Input: part model. Units: mm. Frame: model coordinates. Coordinates: 2 decimals unless noted, no trailing zeros. Order: outer loops, then holes, each group sorted by start corner. A loop starts at its lowest first (then second) coordinate and runs counter-clockwise, first axis right, second up. Notation, with made-up numbers: M 30.25,25 L 68.25,25 A14 ccw 68.25,39 Z; hole C 27.5,64 d8. An arc over 180 degrees is marked long. Answer in a Markdown table with one row per item.
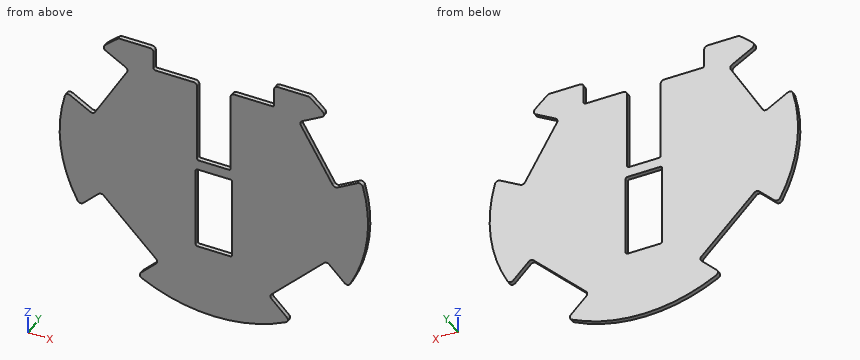
from build123d import *

# Parameters (mm, degrees)
RESSALTO_EXTRUS_O1_DEPTH = 2.5
ESBO_O13_W               = 20.5
ESBO_O13_H               = 48
CORTE_EXTRUS_O8_DEPTH    = 124.061976256
FILETE1_R                = 2
FILETE2_R                = 1


# Read off the part's stored shape, not the designer's step: Ressalto-extrusão1
with BuildPart() as part:
    # Ressalto-extrusão1 outline → Ressalto-extrusão1 (new body)
    with BuildSketch(Plane(origin=(0, 0, 0), x_dir=(1, 0, 0), z_dir=(0, 1, 0))):
        with BuildLine():
            ThreePointArc((41.182170498, 73.709082433), (41.745717904, 75.420720863), (40.703673569, 76.89090296))
            ThreePointArc((40.703673569, 76.89090296), (0, 87), (-40.703673569, 76.89090296))
            ThreePointArc((-40.703673569, 76.89090296), (-41.745717904, 75.420720863), (-41.182170498, 73.709082433))
            Line((-41.182170498, 73.709082433), (-32.526911935, 65.053823869))
            ThreePointArc((-32.526911935, 65.053823869), (-31.941125497, 63.639610306), (-32.526911935, 62.225396744))
            Line((-32.526911935, 62.225396744), (-62.225396744, 32.526911935))
            ThreePointArc((-62.225396744, 32.526911935), (-63.639610306, 31.941125497), (-65.053823869, 32.526911935))
            Line((-65.053823869, 32.526911935), (-73.709082433, 41.182170498))
            ThreePointArc((-73.709082433, 41.182170498), (-75.420720863, 41.745717904), (-76.89090296, 40.703673569))
            ThreePointArc((-76.89090296, 40.703673569), (-86.449685697, 9.769945899), (-84.035651423, -22.516866789))
            ThreePointArc((-84.035651423, -22.516866789), (-82.869168521, -23.846994955), (-81.103797367, -23.731288475))
            Line((-81.103797367, -23.731288475), (-69.755752861, -17.179491924))
            ThreePointArc((-69.755752861, -17.179491924), (-68.238114771, -16.979691079), (-67.023702054, -17.911542732))
            Line((-67.023702054, -17.911542732), (-49.023702054, -49.088457268))
            ThreePointArc((-49.023702054, -49.088457268), (-48.823901209, -50.606095358), (-49.755752861, -51.820508076))
            Line((-49.755752861, -51.820508076), (-61.103797367, -58.372304626))
            ThreePointArc((-61.103797367, -58.372304626), (-62.086687696, -59.843307652), (-61.518004364, -61.518575561))
            ThreePointArc((-61.518004364, -61.518575561), (-57.944854795, -64.895252544), (-54.186675605, -68.064705882))
            ThreePointArc((-54.186675605, -68.064705882), (-53.600773132, -68.388042871), (-52.941004902, -68.5))
            Line((-52.941004902, -68.5), (52.941004902, -68.5))
            ThreePointArc((52.941004902, -68.5), (53.600773132, -68.388042871), (54.186675605, -68.064705882))
            ThreePointArc((54.186675605, -68.064705882), (57.944854795, -64.895252544), (61.518004364, -61.518575561))
            ThreePointArc((61.518004364, -61.518575561), (62.086687696, -59.843307652), (61.103797367, -58.372304626))
            Line((61.103797367, -58.372304626), (49.755752861, -51.820508076))
            ThreePointArc((49.755752861, -51.820508076), (48.823901209, -50.606095358), (49.023702054, -49.088457268))
            Line((49.023702054, -49.088457268), (67.023702054, -17.911542732))
            ThreePointArc((67.023702054, -17.911542732), (68.238114771, -16.979691079), (69.755752861, -17.179491924))
            Line((69.755752861, -17.179491924), (81.103797367, -23.731288475))
            ThreePointArc((81.103797367, -23.731288475), (82.869168521, -23.846994955), (84.035651423, -22.516866789))
            ThreePointArc((84.035651423, -22.516866789), (86.449685697, 9.769945899), (76.89090296, 40.703673569))
            ThreePointArc((76.89090296, 40.703673569), (75.420720863, 41.745717904), (73.709082433, 41.182170498))
            Line((73.709082433, 41.182170498), (65.053823869, 32.526911935))
            ThreePointArc((65.053823869, 32.526911935), (63.639610306, 31.941125497), (62.225396744, 32.526911935))
            Line((62.225396744, 32.526911935), (32.526911935, 62.225396744))
            ThreePointArc((32.526911935, 62.225396744), (31.941125497, 63.639610306), (32.526911935, 65.053823869))
            Line((32.526911935, 65.053823869), (41.182170498, 73.709082433))
        make_face()
    extrude(amount=RESSALTO_EXTRUS_O1_DEPTH)

    # Esboço13 → Corte-extrusão8 (cut, through all)
    with BuildSketch(Plane.XZ):
        with BuildLine():
            ThreePointArc((-9.5, 67.5), (-9.207106781, 68.207106781), (-8.5, 68.5))
            Line((-8.5, 68.5), (-34, 68.5))
            Line((-34, 68.5), (-34, 55.5))
            Line((-34, 55.5), (-9.5, 55.5))
            Line((-9.5, 55.5), (-9.5, 67.5))
        make_face()
        with BuildLine():
            Line((34, 68.5), (8.5, 68.5))
            ThreePointArc((8.5, 68.5), (9.207106781, 68.207106781), (9.5, 67.5))
            Line((9.5, 67.5), (9.5, 55.5))
            Line((9.5, 55.5), (34, 55.5))
            Line((34, 55.5), (34, 68.5))
        make_face()
        with BuildLine():
            Line((8.5, 68.5), (-8.5, 68.5))
            ThreePointArc((-8.5, 68.5), (-9.207106781, 68.207106781), (-9.5, 67.5))
            Line((-9.5, 67.5), (-9.5, 55.5))
            Line((-9.5, 55.5), (9.5, 55.5))
            Line((9.5, 55.5), (9.5, 67.5))
            ThreePointArc((9.5, 67.5), (9.207106781, 68.207106781), (8.5, 68.5))
        make_face()
        with BuildLine():
            Line((9.5, 55.5), (-9.5, 55.5))
            Line((-9.5, 55.5), (-9.5, 8.5))
            ThreePointArc((-9.5, 8.5), (-9.207106781, 7.792893219), (-8.5, 7.5))
            Line((-8.5, 7.5), (8.5, 7.5))
            ThreePointArc((8.5, 7.5), (9.207106781, 7.792893219), (9.5, 8.5))
            Line((9.5, 8.5), (9.5, 55.5))
        make_face()
        with Locations((0, -22.35)):
            Rectangle(ESBO_O13_W, ESBO_O13_H)
    extrude(amount=-CORTE_EXTRUS_O8_DEPTH, mode=Mode.SUBTRACT)

    # Filete1
    filete1_edges = [part.edges().sort_by_distance(p)[0] for p in [
        (-9.5, 1.25, 55.5),
        (-34, 1.25, 68.5),
        (34, 1.25, 68.5),
        (9.5, 1.25, 55.5),
    ]]
    fillet(filete1_edges, radius=FILETE1_R)

    # Filete2
    filete2_edges = [part.edges().sort_by_distance(p)[0] for p in [
        (-34, 1.25, 55.5),
        (34, 1.25, 55.5),
        (-10.25, 1.25, 1.65),
        (10.25, 1.25, 1.65),
        (10.25, 1.25, -46.35),
        (-10.25, 1.25, -46.35),
    ]]
    fillet(filete2_edges, radius=FILETE2_R)


solid = part.part
1) Cut plane D-D, the plane x = 26.5. Output: boundary loops of the cut face in (y, z).
Resolved:
| item | result |
|---|---|
| outline | M 0,-82.87 L 2.5,-82.87 L 2.5,55.5 L 0,55.5 Z |
2) Cut plane B-B, the plane z = -20.5. Output: boundary loops of the cut face in (x, y).
Resolved:
| item | result |
|---|---|
| outline | M -84.55,0 L -10.25,0 L -10.25,2.5 L -84.55,2.5 Z; M 10.25,0 L 84.55,0 L 84.55,2.5 L 10.25,2.5 Z |
3) Contact query for flat-ended pins moving along their axis: pin 1 (10 mm diameter, centred on x = 32.5, z = -58, fed in from -Y); pin 2 (1.5 mm diameter, centred on x = 2, y = 1, fed in from +Z); pin 3 (1.2 mm diameter, centred on y = 1.5, z = 23.5, fed in from +X); pin 4 (1.2 mm diameter, centred on x = 25.5, y = 1.5, fed in from +Z). Output: stop coordinate, or through.
Resolved:
| item | result |
|---|---|
| pin 1 | stops at y = 0 |
| pin 2 | stops at z = 7.5 |
| pin 3 | stops at x = 83.89 |
| pin 4 | stops at z = 55.5 |
4) Cut plane A-A, the plane z = 43. Output: boundary loops of the cut face in (x, y).
Resolved:
| item | result |
|---|---|
| outline | M -52.54,0 L -9.5,0 L -9.5,2.5 L -52.54,2.5 Z; M 9.5,0 L 52.54,0 L 52.54,2.5 L 9.5,2.5 Z |
5) Material intervals for probe 1 along X at (y, z) = (0.35, 21.5); probe 2 along X at (y, z) = (2, -31); probe 3 along X at (y, z) = (1.1, -18), sorted ascending.
Resolved:
| item | result |
|---|---|
| probe 1 | x = -84.3 to -77.24, -64.95 to -9.5, 9.5 to 64.95, 77.24 to 84.3 |
| probe 2 | x = -81.29 to -10.25, 10.25 to 81.29 |
| probe 3 | x = -85.12 to -10.25, 10.25 to 85.12 |
6) Cut plane C-C, the plane x = -23.5. Output: boundary loops of the cut face in (y, z), and give its area (3 significant figures).
Resolved:
| item | result |
|---|---|
| outline | M 0,-83.77 L 2.5,-83.77 L 2.5,55.5 L 0,55.5 Z |
| area | 348 mm2 |
